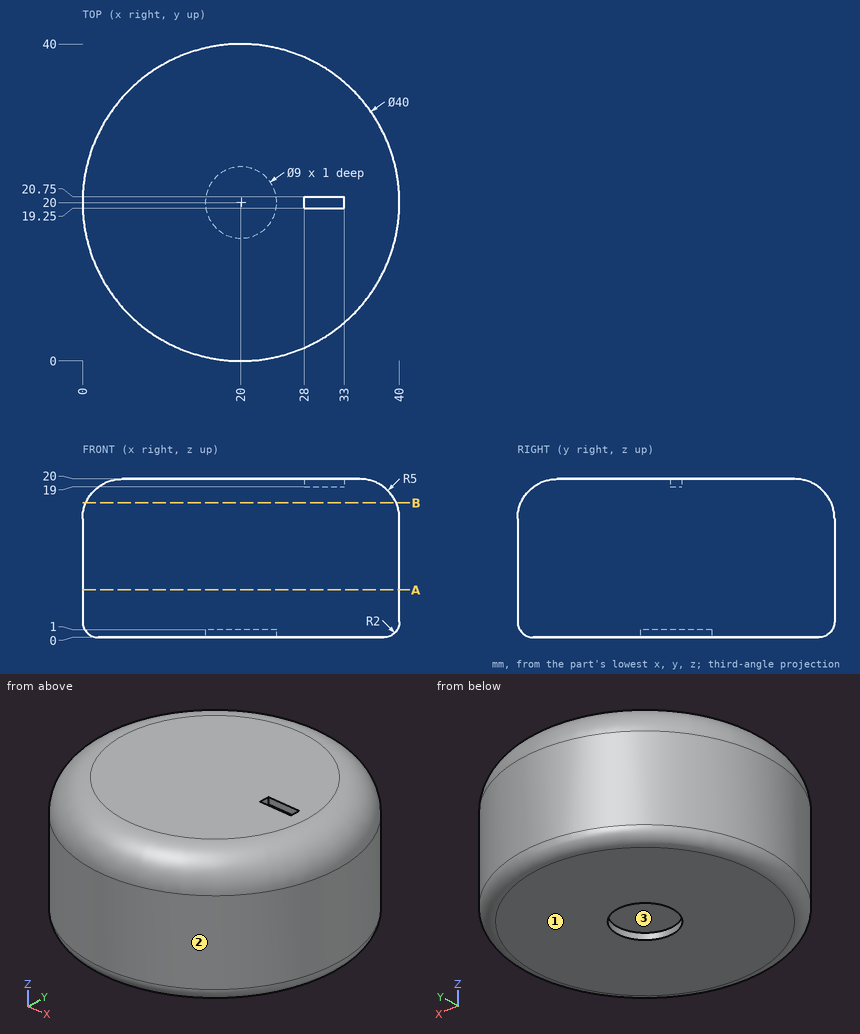
Geometry check sheet. Reference: drawing and pictorial views, mm from the part's lowest x, y, z. Give positions to 0.01 mm unless a question says otherwise; leave off trailing zeros. Write each loop counter-clockwise with the first axis right and the second up, starting at its lowest first coordinate (ties: lowest second). Pieces come first, ordered by that corner, then holes. Notation, with made-up numbers: (1, 39) - (56, 39) arc R21 ccw to (56, 61) - close; hole circle Ø8 at (-25, 47.25). An arc over 180 degrees is marked (long way). Put each result on its own line as item: value.
Q1. Section check B-B on z = 17. Record the cut outline in (x, y), and give its area (3 significant figures).
Result:
outline: circle Ø39.17 at (20, 20)
area: 1,200 mm2
Q2. Mould release check, pull along Y, two halves, no side actions. Record for the marked faces 1, 2 and 3: released by +Y, released by -Y, zero draft, split by the parting line, or undercut.
Result:
face 1: zero draft
face 2: split by the parting line
face 3: undercut
Q3. Depth check by flat-ended pin: P1, Ø8, axis at x = 25.5, z = 12.5, coming from the +Y side; P2, Ø1.1, axis at y = 20.5, z = 19.5, coming from the +X side; P3, Ø4, axis at x = 29, z = 5.5, coming from the +Y side (3 decimals). Enter the tip coordinate at first touch or a pass-through.
Result:
P1: y = 39.94
P2: x = 38.06
P3: y = 38.735
Q4. Scan lines: probe 1 along Y at (x, z) = (20, 0.3); probe 2 along Z at (x, y) = (19.5, 17); probe 3 along Y at (x, z) = (20, 0.8). Record each from-to range of solid material in increasing order. Write a range as from..to.
Result:
probe 1: 0.95..15.5, 24.5..39.05
probe 2: 1..20
probe 3: 0.4..15.5, 24.5..39.6
Q5. Section check A-A on z = 6. Record the cut outline in (x, y).
Result:
outline: circle Ø40 at (20, 20)
